The listing builds one solid part. Answer for the finished solid, in the listing's coordinates (mm). Round coordinates to 2 decimals unless told otherwise and drop trailing zeros. Write each loop counter-clockwise with the first axis right and the second up, starting at its lowest first coordinate (ties: lowest second). Pieces come first, ordered by that corner, then holes. Notation, with made-up numbers: M 87.5,81 L 107.5,81 A13 ccw 107.5,103 Z; hole C -17.5,56 d3. An arc over 180 degrees is marked long. Answer as CSV lines item,"result". Start each with the question number.
from build123d import *

# Parameters (mm, degrees)
SKETCH1_R           = 2.4892
SKETCH1_R_2         = 14.2875
SKETCH1_R_3         = 29.9974
BOSS_EXTRUDE1_DEPTH = 3.175
FILLET1_R           = 10.16


with BuildPart() as part:
    # Sketch1 → Boss-Extrude1 (new body)
    with BuildSketch(Plane.XY):
        Polygon((-152.4, 0), (152.4, 0), (152.4, 116.084254136), (134.559727495, 165.1), (-152.4, 165.1), align=None)
        with Locations((-139.7, 158.75)):
            Circle(SKETCH1_R, mode=Mode.SUBTRACT)
        with Locations((96.278017777, 158.881185382)):
            Circle(SKETCH1_R, mode=Mode.SUBTRACT)
        with Locations((112.555769881, 151.290744918)):
            Circle(SKETCH1_R, mode=Mode.SUBTRACT)
        with Locations((124.489866165, 155.634400739)):
            Circle(SKETCH1_R, mode=Mode.SUBTRACT)
        with Locations((114.3, 69.85)):
            Circle(SKETCH1_R, mode=Mode.SUBTRACT)
        with Locations((127, 69.85)):
            Circle(SKETCH1_R, mode=Mode.SUBTRACT)
        with Locations((139.7, 69.85)):
            Circle(SKETCH1_R, mode=Mode.SUBTRACT)
        with Locations((100.621673597, 146.947089098)):
            Circle(SKETCH1_R, mode=Mode.SUBTRACT)
        with Locations((116.899425702, 139.356648634)):
            Circle(SKETCH1_R, mode=Mode.SUBTRACT)
        with Locations((128.833521986, 143.700304455)):
            Circle(SKETCH1_R, mode=Mode.SUBTRACT)
        with Locations((104.965329418, 135.012992814)):
            Circle(SKETCH1_R, mode=Mode.SUBTRACT)
        with Locations((121.243081522, 127.42255235)):
            Circle(SKETCH1_R, mode=Mode.SUBTRACT)
        with Locations((133.177177806, 131.766208171)):
            Circle(SKETCH1_R, mode=Mode.SUBTRACT)
        with Locations((109.308985238, 123.07889653)):
            Circle(SKETCH1_R, mode=Mode.SUBTRACT)
        with Locations((125.586737342, 115.488456066)):
            Circle(SKETCH1_R, mode=Mode.SUBTRACT)
        with Locations((137.520833626, 119.832111887)):
            Circle(SKETCH1_R, mode=Mode.SUBTRACT)
        with Locations((113.652641058, 111.144800246)):
            Circle(SKETCH1_R, mode=Mode.SUBTRACT)
        with Locations((129.930393162, 103.554359782)):
            Circle(SKETCH1_R, mode=Mode.SUBTRACT)
        with Locations((141.864489446, 107.898015603)):
            Circle(SKETCH1_R, mode=Mode.SUBTRACT)
        with Locations((117.996296878, 99.210703962)):
            Circle(SKETCH1_R, mode=Mode.SUBTRACT)
        with Locations((134.274048982, 91.620263498)):
            Circle(SKETCH1_R, mode=Mode.SUBTRACT)
        with Locations((146.208145266, 95.963919319)):
            Circle(SKETCH1_R, mode=Mode.SUBTRACT)
        with Locations((114.3, 57.15)):
            Circle(SKETCH1_R, mode=Mode.SUBTRACT)
        with Locations((127, 57.15)):
            Circle(SKETCH1_R, mode=Mode.SUBTRACT)
        with Locations((139.7, 57.15)):
            Circle(SKETCH1_R, mode=Mode.SUBTRACT)
        with Locations((114.3, 44.45)):
            Circle(SKETCH1_R, mode=Mode.SUBTRACT)
        with Locations((127, 44.45)):
            Circle(SKETCH1_R, mode=Mode.SUBTRACT)
        with Locations((139.7, 44.45)):
            Circle(SKETCH1_R, mode=Mode.SUBTRACT)
        with Locations((114.3, 31.75)):
            Circle(SKETCH1_R, mode=Mode.SUBTRACT)
        with Locations((127, 31.75)):
            Circle(SKETCH1_R, mode=Mode.SUBTRACT)
        with Locations((139.7, 31.75)):
            Circle(SKETCH1_R, mode=Mode.SUBTRACT)
        with Locations((114.3, 19.05)):
            Circle(SKETCH1_R, mode=Mode.SUBTRACT)
        with Locations((127, 19.05)):
            Circle(SKETCH1_R, mode=Mode.SUBTRACT)
        with Locations((139.7, 19.05)):
            Circle(SKETCH1_R, mode=Mode.SUBTRACT)
        with Locations((114.3, 6.35)):
            Circle(SKETCH1_R, mode=Mode.SUBTRACT)
        with Locations((127, 6.35)):
            Circle(SKETCH1_R, mode=Mode.SUBTRACT)
        with Locations((139.7, 6.35)):
            Circle(SKETCH1_R, mode=Mode.SUBTRACT)
        with Locations((-127, 158.75)):
            Circle(SKETCH1_R, mode=Mode.SUBTRACT)
        with Locations((-114.3, 158.75)):
            Circle(SKETCH1_R, mode=Mode.SUBTRACT)
        with Locations((-127, 146.05)):
            Circle(SKETCH1_R, mode=Mode.SUBTRACT)
        with Locations((-114.3, 146.05)):
            Circle(SKETCH1_R, mode=Mode.SUBTRACT)
        with Locations((-127, 133.35)):
            Circle(SKETCH1_R, mode=Mode.SUBTRACT)
        with Locations((-114.3, 133.35)):
            Circle(SKETCH1_R, mode=Mode.SUBTRACT)
        with Locations((-127, 120.65)):
            Circle(SKETCH1_R, mode=Mode.SUBTRACT)
        with Locations((-114.3, 120.65)):
            Circle(SKETCH1_R, mode=Mode.SUBTRACT)
        with Locations((-127, 107.95)):
            Circle(SKETCH1_R, mode=Mode.SUBTRACT)
        with Locations((-114.3, 107.95)):
            Circle(SKETCH1_R, mode=Mode.SUBTRACT)
        with Locations((-127, 95.25)):
            Circle(SKETCH1_R, mode=Mode.SUBTRACT)
        with Locations((-114.3, 95.25)):
            Circle(SKETCH1_R, mode=Mode.SUBTRACT)
        with Locations((-127, 82.55)):
            Circle(SKETCH1_R, mode=Mode.SUBTRACT)
        with Locations((-114.3, 82.55)):
            Circle(SKETCH1_R, mode=Mode.SUBTRACT)
        with Locations((-127, 69.85)):
            Circle(SKETCH1_R, mode=Mode.SUBTRACT)
        with Locations((-114.3, 69.85)):
            Circle(SKETCH1_R, mode=Mode.SUBTRACT)
        with Locations((-127, 57.15)):
            Circle(SKETCH1_R, mode=Mode.SUBTRACT)
        with Locations((-114.3, 57.15)):
            Circle(SKETCH1_R, mode=Mode.SUBTRACT)
        with Locations((-127, 44.45)):
            Circle(SKETCH1_R, mode=Mode.SUBTRACT)
        with Locations((-114.3, 44.45)):
            Circle(SKETCH1_R, mode=Mode.SUBTRACT)
        with Locations((-127, 31.75)):
            Circle(SKETCH1_R, mode=Mode.SUBTRACT)
        with Locations((-114.3, 31.75)):
            Circle(SKETCH1_R, mode=Mode.SUBTRACT)
        with Locations((-127, 19.05)):
            Circle(SKETCH1_R, mode=Mode.SUBTRACT)
        with Locations((-114.3, 19.05)):
            Circle(SKETCH1_R, mode=Mode.SUBTRACT)
        with Locations((-127, 6.35)):
            Circle(SKETCH1_R, mode=Mode.SUBTRACT)
        with Locations((-114.3, 6.35)):
            Circle(SKETCH1_R, mode=Mode.SUBTRACT)
        with Locations((-139.7, 146.05)):
            Circle(SKETCH1_R, mode=Mode.SUBTRACT)
        with Locations((-139.7, 133.35)):
            Circle(SKETCH1_R, mode=Mode.SUBTRACT)
        with Locations((-139.7, 120.65)):
            Circle(SKETCH1_R, mode=Mode.SUBTRACT)
        with Locations((-139.7, 107.95)):
            Circle(SKETCH1_R, mode=Mode.SUBTRACT)
        with Locations((-139.7, 95.25)):
            Circle(SKETCH1_R, mode=Mode.SUBTRACT)
        with Locations((-139.7, 82.55)):
            Circle(SKETCH1_R, mode=Mode.SUBTRACT)
        with Locations((-139.7, 69.85)):
            Circle(SKETCH1_R, mode=Mode.SUBTRACT)
        with Locations((-139.7, 57.15)):
            Circle(SKETCH1_R, mode=Mode.SUBTRACT)
        with Locations((-139.7, 44.45)):
            Circle(SKETCH1_R, mode=Mode.SUBTRACT)
        with Locations((-139.7, 31.75)):
            Circle(SKETCH1_R, mode=Mode.SUBTRACT)
        with Locations((-139.7, 19.05)):
            Circle(SKETCH1_R, mode=Mode.SUBTRACT)
        with Locations((-139.7, 6.35)):
            Circle(SKETCH1_R, mode=Mode.SUBTRACT)
        with Locations((14.747605731, 115.915231493)):
            Circle(SKETCH1_R_2, mode=Mode.SUBTRACT)
        with Locations((-35.124454019, 66.937360953)):
            Circle(SKETCH1_R_2, mode=Mode.SUBTRACT)
        with Locations((16.872346339, 55.177887184)):
            Circle(SKETCH1_R_2, mode=Mode.SUBTRACT)
        with Locations((62.683226079, 82.500385193)):
            Circle(SKETCH1_R_2, mode=Mode.SUBTRACT)
        with Locations((-64.43319304, 101.664655725)):
            Circle(SKETCH1_R_3, mode=Mode.SUBTRACT)
        with Locations((-64.43319304, 32.068655725)):
            Circle(SKETCH1_R_3, mode=Mode.SUBTRACT)
        with Locations((-5.591406845, 131.129848394)):
            Circle(SKETCH1_R, mode=Mode.SUBTRACT)
        with Locations((35.086618307, 100.700614592)):
            Circle(SKETCH1_R, mode=Mode.SUBTRACT)
        with Locations((-1.212453661, 24.647087184)):
            Circle(SKETCH1_R, mode=Mode.SUBTRACT)
        with Locations((34.957146339, 24.647087184)):
            Circle(SKETCH1_R, mode=Mode.SUBTRACT)
        with Locations((34.957146339, 85.708687184)):
            Circle(SKETCH1_R, mode=Mode.SUBTRACT)
        with Locations((-1.212453661, 85.708687184)):
            Circle(SKETCH1_R, mode=Mode.SUBTRACT)
    extrude(amount=BOSS_EXTRUDE1_DEPTH)

    # Fillet1
    fillet1_edges = [part.edges().sort_by_distance(p)[0] for p in [
        (-152.4, 165.1, 1.5875),
        (134.559727495, 165.1, 1.5875),
        (152.4, 116.084254136, 1.5875),
        (152.4, 0, 1.5875),
        (-152.4, 0, 1.5875),
    ]]
    fillet(fillet1_edges, radius=FILLET1_R)


solid = part.part
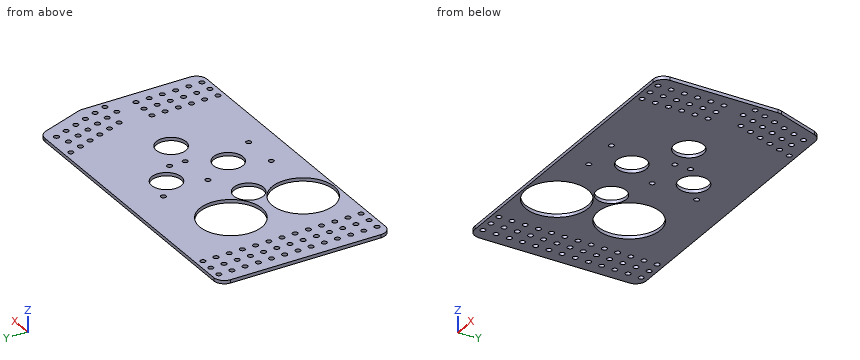
Q1. Find section C-C (z = 2.65). Count the separate pieces of the cut face and the enclosed holes in it, plus the area to 3 significant figures.
Q2. Find section A-A (x = 20.5). Determine the outline of the cut face in (y, z) (3 decimals), plus the area to 3 significant figures.
Q3. Straight lines are drawn through the part: L1, parallel to Y at x = -51, z = 2.25; L2, parallel to X at y = 54, z = 1.15; L3, parallel to Y at x = 109, z = 2.8. For each, find the intervals that lie inside material, in ascending order.
Q4. Find section B-B (x = -31.5). Determine the outline of the cut face in (y, z) (1 decimal), plus the area to 3 significant figures.
Q5. Find section D-D (x = -85). Determine the outline of the cut face in (y, z) (3 decimals), plus the area to 3 significant figures.
Q6. This flat-tipped pin is pushed along its axis until it touches: P1, Ø3, axis at x = 127, y = 19.05, coming from the +Z side. Where does it stop, or does it pass through?
Reported:
1,separate pieces,"1"
1,enclosed holes,"87"
1,area,"40,000 mm2"
2,outline,"M 0,0 L 41.359,0 L 41.359,3.175 L 0,3.175 Z; M 68.997,0 L 102.837,0 L 102.837,3.175 L 68.997,3.175 Z; M 128.994,0 L 165.1,0 L 165.1,3.175 L 128.994,3.175 Z"
2,area,"353 mm2"
3,L1,"y = 0 to 5.25, 58.89 to 74.84, 128.49 to 165.1"
3,L2,"x = -152.4 to -84.9, -43.97 to -41.19, -29.06 to 2.63, 31.11 to 152.4"
3,L3,"y = 0 to 120.61, 125.55 to 165.1"
4,outline,"M 0,0 L 53.1,0 L 53.1,3.2 L 0,3.2 Z; M 80.8,0 L 165.1,0 L 165.1,3.2 L 80.8,3.2 Z"
4,area,"436 mm2"
5,outline,"M 0,0 L 10.232,0 L 10.232,3.175 L 0,3.175 Z; M 53.906,0 L 79.828,0 L 79.828,3.175 L 53.906,3.175 Z; M 123.502,0 L 165.1,0 L 165.1,3.175 L 123.502,3.175 Z"
5,area,"247 mm2"
6,P1,"passes through"
